```python
from build123d import *

# Parameters (mm, degrees)
SKETCH1_R           = 38.1
BOSS_EXTRUDE1_DEPTH = 12.7
SKETCH2_R           = 11.43
BOSS_EXTRUDE2_DEPTH = 73.914
FILLET1_R           = 1.27
FILLET2_R           = 1.27
FILLET3_R           = 3.81
CUT_EXTRUDE1_DEPTH  = 4.445
CUT_EXTRUDE2_DEPTH  = 3.175


with BuildPart() as part:
    # Sketch1 → Boss-Extrude1 (new body)
    with BuildSketch(Plane(origin=(0, 0, 0), x_dir=(1, 0, 0), z_dir=(0, 1, 0))):
        with Locations(Location((0, 0, 0), (0, 0, 270))):
            Circle(SKETCH1_R)
    extrude(amount=BOSS_EXTRUDE1_DEPTH)

    # Sketch2 → Boss-Extrude2 (add)
    with BuildSketch(Plane(origin=(0, 12.7, 0), x_dir=(1, 0, 0), z_dir=(0, 1, 0))):
        with Locations(Location((0, 0, 0), (0, 0, 270))):
            Circle(SKETCH2_R)
    extrude(amount=BOSS_EXTRUDE2_DEPTH)

    # Fillet1
    fillet1_edges = [part.edges().sort_by_distance(p)[0] for p in [
        (0, 12.7, -38.1),
    ]]
    fillet(fillet1_edges, radius=FILLET1_R)

    # Fillet2
    fillet2_edges = [part.edges().sort_by_distance(p)[0] for p in [
        (0, 0, -38.1),
    ]]
    fillet(fillet2_edges, radius=FILLET2_R)

    # Fillet3
    fillet3_edges = [part.edges().sort_by_distance(p)[0] for p in [
        (0, 86.614, -11.43),
    ]]
    fillet(fillet3_edges, radius=FILLET3_R)

    # Sketch4 → Cut-Extrude1 (cut)
    with BuildSketch(Plane(origin=(0, 12.7, 0), x_dir=(1, 0, 0), z_dir=(0, 1, 0))):
        with BuildLine():
            ThreePointArc((-32.279166667, 2.616032168), (-30.612356486, -3.172240023), (-28.469166667, 2.457066199))
            ThreePointArc((-28.469166667, 2.457066199), (-25.354072576, 13.179591374), (-18.367655947, 21.889719962))
            ThreePointArc((-18.367655947, 21.889719962), (-18.132851679, 24.573545023), (-20.81667674, 24.80834929))
            ThreePointArc((-20.81667674, 24.80834929), (-28.773544821, 14.861740929), (-32.279166667, 2.616032168))
        make_face()
        with BuildLine():
            ThreePointArc((32.279166667, -2.616032168), (30.612356486, 3.172240023), (28.469166667, -2.457066199))
            ThreePointArc((28.469166667, -2.457066199), (25.354072576, -13.179591374), (18.367655947, -21.889719962))
            ThreePointArc((18.367655947, -21.889719962), (18.132851679, -24.573545023), (20.81667674, -24.80834929))
            ThreePointArc((20.81667674, -24.80834929), (28.773544821, -14.861740929), (32.279166667, -2.616032168))
        make_face()
    extrude(amount=-CUT_EXTRUDE1_DEPTH, mode=Mode.SUBTRACT)

    # Sketch5 → Cut-Extrude2 (cut)
    with BuildSketch(Plane(origin=(0, 8.255, 0), x_dir=(1, 0, 0), z_dir=(0, 1, 0))):
        with BuildLine():
            ThreePointArc((-21.633017004, 25.781225733), (-30.501788573, 14.223217599), (-33.655, 0))
            ThreePointArc((-33.655, 0), (-30.48, -3.175), (-27.305, 0))
            ThreePointArc((-27.305, 0), (-24.746734125, 11.539591637), (-17.551315682, 20.916843519))
            ThreePointArc((-17.551315682, 20.916843519), (-17.159975236, 25.389885287), (-21.633017004, 25.781225733))
        make_face()
        with BuildLine():
            ThreePointArc((33.655, 0), (30.48, 3.175), (27.305, 0))
            ThreePointArc((27.305, 0), (24.746734125, -11.539591637), (17.551315682, -20.916843519))
            ThreePointArc((17.551315682, -20.916843519), (17.159975236, -25.389885287), (21.633017004, -25.781225733))
            ThreePointArc((21.633017004, -25.781225733), (30.501788573, -14.223217599), (33.655, 0))
        make_face()
    extrude(amount=-CUT_EXTRUDE2_DEPTH, mode=Mode.SUBTRACT)


solid = part.part
```
The model under review builds one solid part; all positions refer to its coordinate system, in mm. A direction names the side the tool comes from. Coordinates: 2 decimals unless noted, no trailing zeros. Write each loop counter-clockwise with the first axis right and the second up, starting at its lowest first coordinate (ties: lowest second). Pieces come first, ordered by that corner, then holes.
1) The part is to be moulded in two halves that separate along X. For faces 4 (the face through (-23.183, 6.279, -30.235)), 5 (the face through (27, 5.08, 11)), 6 (the face through (1, 0, -1)), say which applies: pulls with the +X half, pulls with the -X half, needs draft (parallel to the pull), parting line crosses it, or undercut.
2) Clearance check with flat-ended pins moving along their axes: pin 1 Ø5 at (x, z) = (28.5, 12) entering from +Y; pin 2 Ø10 at (x, y) = (21.5, 12.5) entering from -Z; pin 3 Ø8 at (y, z) = (23.5, 13.5) entering from -X. State where each tip first meets the part, or that it passes through.
3) To check wall thickness, follow probe 1 along X at (y, z) = (11.35, 0) (3 decimals); probe 2 along Y at (x, z) = (-18, -27); probe 3 along X at (y, z) = (10, -4.5). State the ranges of each line that lie inside material, in increasing order.
4) Machinability: for faces 1 (the face through (18.106, 10.509, 24.541)), 2 (the face through (0, 86.614, 0)), 3 (the face through (-24, 8.255, -14)), which of the approach directions +Z, -Z, +X, -X, +Y, -Y give a long, thin tool a straight path to every point of the face, cutting with its end or side? Answer none if there is none.
5) We need section B-B on y = 41. State the section outline as (x, z) points, then the cut area to 3 significant figures.
6) We need section A-A on x = 0. State the section outline as (y, z) points, then the cut area to 3 significant figures.
Answer list:
1. face 4: parting line crosses it
1. face 5: undercut
1. face 6: needs draft
2. pin 1: stops at y = 12.7
2. pin 2: stops at z = -34.29
2. pin 3: stops at x = -6.36
3. probe 1: x = -38.1 to -33.655, -27.305 to 27.305, 33.655 to 38.1
3. probe 2: y = 0 to 12.7
3. probe 3: x = -37.83 to -32.07, -28.22 to 37.83
4. face 1: +Y
4. face 2: +Z, -Z, +X, -X, +Y
4. face 3: none
5. outline: circle Ø22.86 at (0, 0)
5. area: 410 mm2
6. outline: (0, -36.83) arc R1.27 ccw to (1.27, -38.1) - (11.43, -38.1) arc R1.27 ccw to (12.7, -36.83) - (12.7, -11.43) - (82.8, -11.43) arc R3.81 ccw to (86.61, -7.62) - (86.61, 7.62) arc R3.81 ccw to (82.8, 11.43) - (12.7, 11.43) - (12.7, 36.83) arc R1.27 ccw to (11.43, 38.1) - (1.27, 38.1) arc R1.27 ccw to (0, 36.83) - close
6. area: 2,650 mm2
